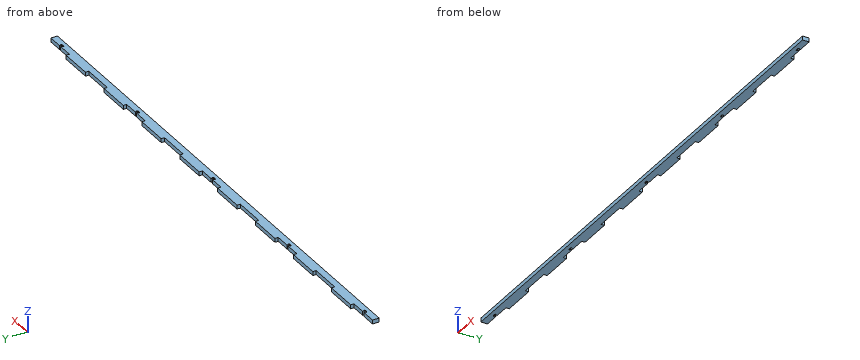
```python
from build123d import *

# Parameters (mm, degrees)
SZKIC1_W                    = 830
SZKIC1_H                    = 16
DODANIE_WYCI_GNI_CIE1_DEPTH = 6
SZKIC2_W                    = 47.778
SZKIC2_H                    = 6
WYTNIJ_WYCI_GNI_CIE1_DEPTH  = 6
SZYK_LINIOWY1_COUNT         = 9
SZYK_LINIOWY1_PITCH         = 97.778
WYTNIJ_WYCI_GNI_CIE2_DEPTH  = 6
SZYK_LINIOWY2_COUNT         = 5
SZYK_LINIOWY2_PITCH         = 195.56
SZKIC5_W                    = 734.446
SZKIC5_H                    = 1
WYTNIJ_WYCI_GNI_CIE3_DEPTH  = 10


with BuildPart() as part:
    # Szkic1 → Dodanie-wyciągnięcie1 (new body)
    with BuildSketch(Plane.XY):
        with Locations((415, 8)):
            Rectangle(SZKIC1_W, SZKIC1_H)
    extrude(amount=DODANIE_WYCI_GNI_CIE1_DEPTH)

    # Szkic2 → Wytnij-wyciągnięcie1 (cut)
    with BuildSketch(Plane(origin=(0, 16, 0), x_dir=(1, 0, 0), z_dir=(0, 1, 0))):
        with Locations((806.111, -3)):
            Rectangle(SZKIC2_W, SZKIC2_H)
    wytnij_wyci_gni_cie1 = extrude(amount=-WYTNIJ_WYCI_GNI_CIE1_DEPTH, mode=Mode.SUBTRACT)

    # Szyk liniowy1: Wytnij-wyciągnięcie1 ×9
    with Locations(*[(-i * SZYK_LINIOWY1_PITCH, 0, 0) for i in range(1, SZYK_LINIOWY1_COUNT)]):
        add(wytnij_wyci_gni_cie1, mode=Mode.SUBTRACT)

    # Szkic4 → Wytnij-wyciągnięcie2 (cut)
    with BuildSketch(Plane.XY.offset(6)):
        Polygon((22.34, 10), (25.44, 10), (25.44, 8), (26.815, 8), (26.815, 6), (25.44, 6), (25.44, 5.5), (22.34, 5.5), (22.34, 6), (20.965, 6), (20.965, 8), (22.34, 8), align=None)
    wytnij_wyci_gni_cie2 = extrude(amount=-WYTNIJ_WYCI_GNI_CIE2_DEPTH, mode=Mode.SUBTRACT)

    # Szyk liniowy2: Wytnij-wyciągnięcie2 ×5
    with Locations(*[(i * SZYK_LINIOWY2_PITCH, 0, 0) for i in range(1, SZYK_LINIOWY2_COUNT)]):
        add(wytnij_wyci_gni_cie2, mode=Mode.SUBTRACT)

    # Szkic5 → Wytnij-wyciągnięcie3 (cut)
    with BuildSketch(Plane.XY.offset(6)):
        with Locations((414.999, 15.5)):
            Rectangle(SZKIC5_W, SZKIC5_H)
    extrude(amount=-WYTNIJ_WYCI_GNI_CIE3_DEPTH, mode=Mode.SUBTRACT)


solid = part.part
```
Work out the finished part from the listing and answer in its coordinate system (mm). Round coordinates to 2 decimals unless told otherwise and drop trailing zeros. Write each loop counter-clockwise with the first axis right and the second up, starting at its lowest first coordinate (ties: lowest second). Pieces come first, ordered by that corner, then holes. Notation, with made-up numbers: (-7.75, -38.5) - (21.25, -38.5) arc R18 ccw to (21.25, -31.5) - close; hole circle Ø4 at (57.5, -12). An arc over 180 degrees is marked (long way). Return JSON: item names as keys, results as strings. Group by question number.
Q1. Each of these flat-tipped pins is pushed along its axis until it touches: pin 1 Ø1.8 at (x, z) = (792.5, 4) entering from +Y; pin 2 Ø2.5 at (y, z) = (12, 2.5) entering from -X; pin 3 Ø1.5 at (y, z) = (13, 4) entering from +X. Where does it stop, or does it pass through?
Q2. Find the intervals of material crossed by L1, parallel to X at y = 7.25, z = 3.75 (3 decimals); L2, parallel to Y at x = 783.5, z = 1.5, in increasing order.
Q3. The part is cut by section A-A on x = 209.5. Write down the section's boundary in (y, z), then the cut area to 3 significant figures.
Solved:
{
 "1": {"pin 1": "y = 10", "pin 2": "x = 47.78", "pin 3": "x = 782.22"},
 "2": {"L1": "0 to 20.965, 26.815 to 216.525, 222.375 to 412.085, 417.935 to 607.645, 613.495 to 803.205, 809.055 to 830", "L2": "0 to 10"},
 "3": {"outline": "(0, 0) - (10, 0) - (10, 6) - (0, 6) - close", "area": "60.0 mm²"}
}
